Geometry check sheet. Reference: the model listing, model coordinates, mm. A direction names the side the tool comes from. Round coordinates to 2 decimals unless told otherwise and drop trailing zeros. Order: outer loops, then holes, each group sorted by start corner. A loop starts at its lowest first (then second) coordinate and runs counter-clockwise, first axis right, second up. Notation, with made-up numbers: (56.25, 45.5) - (85.25, 45.5) arc R11 cw to (85.25, 59.5) - close; hole circle Ø5 at (26, -14). An arc over 180 degrees is marked (long way). Return JSON: item names as keys, results as strings. Group by question number.
Q1. Sectioned sample at A-A, the plane z = 18. Record the cut outline in (x, y).
Q2. Tool access check on faces 1 (the flat face through (3, 19, 31)), 2 (the flat face through (0, 19, 31)). Record the directions out of +Z, -Z, +X, -X, +Y, -Y that give a thin tool (end or side, any length) a straight path to the whole face; none if there is none.
Q3. Sectioned sample at B-B, the plane x = 990. Record the cut outline in (y, z), then the cut area to 3 significant figures.
Q4. Material ranges on line 1 along X through (y, z) = (32, 51.5); line 2 along Y through (x, z) = (278, 33); line 3 along X through (y, z) = (14, 45), recorded low to high.
Q5. Gauge pin test, flat ends, axial feed: pin 1 Ø4 at (x, y) = (628, 32.5) entering from +Z; pin 2 Ø6.5 at (x, z) = (1617.5, 49.5) entering from -Y; pin 3 Ø7.5 at (x, y) = (27.5, 19.5) entering from +Z; pin 4 Ø1.5 at (x, y) = (476, 18.5) entering from -Z. Record the tip position at first contact, or that the pin passes through.
Q6. Draft check along Z on faces 3 (the flat face through (806, 19, 0)), 4 (the flat face through (1632, 19, 31)), 5 (the flat face through (1635, 19, 31)). Enter one of: pulls with the +Z half, pulls with the -Z half, needs draft (parallel to the pull), parting line crosses it, or undercut.
```python
from build123d import *

# Parameters (mm, degrees)
SKETCH1_W            = 1635
SKETCH1_H            = 38
BOSS_EXTRUDE1_DEPTH  = 62
SKETCH2_W            = 1615
SKETCH2_H            = 38
CUT_EXTRUDE1_DEPTH   = 25
SKETCH3_W            = 18.796
SKETCH3_H            = 15.494
BOSS_EXTRUDE2_DEPTH  = 30.226
SKETCH5_W            = 18.91876422
SKETCH5_H            = 15.494
BOSS_EXTRUDE3_DEPTH  = 30.226
SKETCH6_R            = 3
CUT_EXTRUDE2_DEPTH   = 10
SKETCH7_R            = 3
CUT_EXTRUDE3_DEPTH   = 10
SHELL1_START         = 3
SHELL1_OUTLINE_W     = 32
SHELL1_OUTLINE_H     = 34
SHELL1_DEPTH         = 1629
SHELL1_START_2       = 1607.774
SHELL1_2_OUTLINE_W   = 9.494
SHELL1_2_OUTLINE_H   = 12.91876422
SHELL1_2_DEPTH       = 24.226
SHELL1_3_OUTLINE_W   = 9.494
SHELL1_3_OUTLINE_H   = 12.796
SHELL1_3_DEPTH       = 24.226
SHELL1_4_OUTLINE_W   = 32
SHELL1_4_OUTLINE_H   = 22
SHELL1_4_OUTLINE_W_2 = 9.494
SHELL1_4_OUTLINE_H_2 = 12.796
SHELL1_4_DEPTH       = 4
SHELL1_START_3       = 1628
SHELL1_5_OUTLINE_W   = 32
SHELL1_5_OUTLINE_H   = 22
SHELL1_5_OUTLINE_W_2 = 9.494
SHELL1_5_OUTLINE_H_2 = 12.91876422
SHELL1_5_DEPTH       = 4
SHELL1_START_4       = 1597.774
SHELL1_6_DEPTH       = 10
SHELL1_START_5       = 27.226
SHELL1_7_DEPTH       = 10


# Read off the part's stored shape, not the designer's step: Shell1
with BuildPart() as part:
    # Sketch1 → Boss-Extrude1 (new body)
    with BuildSketch(Plane.XY):
        with Locations((817.5, 19)):
            Rectangle(SKETCH1_W, SKETCH1_H)
    extrude(amount=BOSS_EXTRUDE1_DEPTH)

    # Sketch2 → Cut-Extrude1 (cut)
    with BuildSketch(Plane.XY.offset(62)):
        with Locations((817.5, 19)):
            Rectangle(SKETCH2_W, SKETCH2_H)
    extrude(amount=-CUT_EXTRUDE1_DEPTH, mode=Mode.SUBTRACT)

    # Sketch3 → Boss-Extrude2 (add)
    with BuildSketch(Plane(origin=(10, 0, 0), x_dir=(0, 0, -1), z_dir=(1, 0, 0))):
        with Locations((-49.502, 18.998)):
            Rectangle(SKETCH3_W, SKETCH3_H)
    extrude(amount=BOSS_EXTRUDE2_DEPTH)

    # Sketch5 → Boss-Extrude3 (add)
    with BuildSketch(Plane.ZY.offset(-1625)):
        with Locations((49.44061789, 18.993)):
            Rectangle(SKETCH5_W, SKETCH5_H)
    extrude(amount=BOSS_EXTRUDE3_DEPTH)

    # Sketch6 → Cut-Extrude2 (cut)
    with BuildSketch(Plane(origin=(40.226, 0, 0), x_dir=(0, 0, -1), z_dir=(1, 0, 0))):
        with Locations((-49.504, 18.996)):
            Circle(SKETCH6_R)
    extrude(amount=-CUT_EXTRUDE2_DEPTH, mode=Mode.SUBTRACT)

    # Sketch7 → Cut-Extrude3 (cut)
    with BuildSketch(Plane.ZY.offset(-1594.774)):
        with Locations((49.38123578, 18.995)):
            Circle(SKETCH7_R)
    extrude(amount=-CUT_EXTRUDE3_DEPTH, mode=Mode.SUBTRACT)

    # Shell1 outline → Shell1 (cut)
    with BuildSketch(Plane.YZ.offset(SHELL1_START)):
        with Locations((19, 20)):
            Rectangle(SHELL1_OUTLINE_W, SHELL1_OUTLINE_H)
    extrude(amount=SHELL1_DEPTH, mode=Mode.SUBTRACT)

    # Shell1 2 outline → Shell1 2 (cut)
    with BuildSketch(Plane.YZ.offset(SHELL1_START_2)):
        with Locations((18.993, 49.44061789)):
            Rectangle(SHELL1_2_OUTLINE_W, SHELL1_2_OUTLINE_H)
    extrude(amount=SHELL1_2_DEPTH, mode=Mode.SUBTRACT)

    # Shell1 3 outline → Shell1 3 (cut)
    with BuildSketch(Plane.YZ.offset(SHELL1_START)):
        with Locations((18.998, 49.502)):
            Rectangle(SHELL1_3_OUTLINE_W, SHELL1_3_OUTLINE_H)
    extrude(amount=SHELL1_3_DEPTH, mode=Mode.SUBTRACT)

    # Shell1 4 outline → Shell1 4 (cut)
    with BuildSketch(Plane.YZ.offset(SHELL1_START)):
        with Locations((19, 48)):
            Rectangle(SHELL1_4_OUTLINE_W, SHELL1_4_OUTLINE_H)
        with Locations((18.998, 49.502)):
            Rectangle(SHELL1_4_OUTLINE_W_2, SHELL1_4_OUTLINE_H_2, mode=Mode.SUBTRACT)
    extrude(amount=SHELL1_4_DEPTH, mode=Mode.SUBTRACT)

    # Shell1 5 outline → Shell1 5 (cut)
    with BuildSketch(Plane.YZ.offset(SHELL1_START_3)):
        with Locations((19, 48)):
            Rectangle(SHELL1_5_OUTLINE_W, SHELL1_5_OUTLINE_H)
        with Locations((18.993, 49.44061789)):
            Rectangle(SHELL1_5_OUTLINE_W_2, SHELL1_5_OUTLINE_H_2, mode=Mode.SUBTRACT)
    extrude(amount=SHELL1_5_DEPTH, mode=Mode.SUBTRACT)

    # Shell1 6 outline → Shell1 6 (cut)
    with BuildSketch(Plane.YZ.offset(SHELL1_START_4)):
        with BuildLine():
            Line((23.74, 55.9), (14.246, 55.9))
            Line((14.246, 55.9), (14.246, 53.048250779))
            ThreePointArc((14.246, 53.048250779), (18.991729891, 55.381234889), (23.74, 53.053425182))
            Line((23.74, 53.053425182), (23.74, 55.9))
        make_face()
        with BuildLine():
            ThreePointArc((23.74, 45.709046379), (18.991729891, 43.381236672), (14.246, 45.714220782))
            Line((14.246, 45.714220782), (14.246, 42.98123578))
            Line((14.246, 42.98123578), (23.74, 42.98123578))
            Line((23.74, 42.98123578), (23.74, 45.709046379))
        make_face()
    extrude(amount=SHELL1_6_DEPTH, mode=Mode.SUBTRACT)

    # Shell1 7 outline → Shell1 7 (cut)
    with BuildSketch(Plane.YZ.offset(SHELL1_START_5)):
        with BuildLine():
            Line((23.745, 53.171014999), (23.745, 55.9))
            Line((23.745, 55.9), (14.251, 55.9))
            Line((14.251, 55.9), (14.251, 53.176189401))
            ThreePointArc((14.251, 53.176189401), (18.999270109, 55.503999109), (23.745, 53.171014999))
        make_face()
        with BuildLine():
            Line((23.745, 43.104), (23.745, 45.836985001))
            ThreePointArc((23.745, 45.836985001), (18.999270109, 43.504000891), (14.251, 45.831810599))
            Line((14.251, 45.831810599), (14.251, 43.104))
            Line((14.251, 43.104), (23.745, 43.104))
        make_face()
    extrude(amount=SHELL1_7_DEPTH, mode=Mode.SUBTRACT)


solid = part.part
```
Reply:
{
 "1": {"outline": "(0, 0) - (1635, 0) - (1635, 38) - (0, 38) - close; hole (3, 3) - (1632, 3) - (1632, 35) - (3, 35) - close"},
 "2": {"face 1": "none", "face 2": "+Z, -Z, -X, +Y, -Y"},
 "3": {"outline": "(0, 0) - (38, 0) - (38, 37) - (35, 37) - (35, 3) - (3, 3) - (3, 37) - (0, 37) - close", "area": "318 mm^2"},
 "4": {"line 1": "0 to 3, 7 to 10, 1625 to 1628, 1632 to 1635", "line 2": "0 to 3, 35 to 38", "line 3": "0 to 3, 7 to 40.23, 1594.77 to 1628, 1632 to 1635"},
 "5": {"pin 1": "z = 3", "pin 2": "y = 11.25", "pin 3": "z = 58.9", "pin 4": "z = 0"},
 "6": {"face 3": "pulls with the -Z half", "face 4": "undercut", "face 5": "needs draft"}
}
